Check sheet for the modelled part. Datum: model origin and axes. Units: mm. A direction names the side the tool comes from. Give positions to 0.01 mm unless a question says otherwise; leave off trailing zeros. Order: outer loops, then holes, each group sorted by start corner. A loop starts at its lowest first (then second) coordinate and runs counter-clockwise, first axis right, second up.
Item 1: Access from +Z, -Z, +X, -X, +Y, -Y to the whole of each face (thin tool, end or side, straight path). Record for faces 4 (the flat face through (7.5, 4.8, 0.7)), 5 (the flat face through (-3, 3, 0)), 6 (the flat face through (0, 8, -50)), 7 (the flat face through (0, 14, 10)), 8 (the flat face through (-5, 5, -1)).
Item 2: Sectioned sample at A-A on z = -23.5. Record the boundary of the cut face in (x, y), and give its area (3 significant figures).
Item 3: Gauge pin test, flat end, axial feed: P1, Ø7, axis at x = 0, z = 0, coming from the +Y side. Record the tip position at first contact, or that the pin passes through.
Item 4: Release check for a two-part mould opening along Z. For faces 1 (the flat face through (3, 0, 1)), 2 (the flat face through (0, 15, -10)), 3 (the flat face through (-0.1, 1.3, 48.8)) record: released by +Z, released by -Z, zero draft, split by the parting line, or undercut.
Item 5: Sectioned sample at D-D on z = 0. Record the boundary of the cut face in (x, y), and give its area (3 significant figures).
Item 6: Material ranges on line 1 along Y through (x, z) = (-1, 30); line 2 along Z through (x, y) = (0.75, 7.5); line 3 along Z through (x, y) = (1, 13.25), recorded low to high.
Item 7: Sectioned sample at B-B on y = 15.75. Record the boundary of the cut face in (x, z), and give its area (3 significant figures).
Item 8: Sectioned sample at C-C on x = 0. Record the boundary of the cut face in (y, z), and give its area (4 significant figures).
from build123d import *

# Parameters (mm, degrees)
BOSS_EXTRUDE1_DEPTH = 7.5
CHAMFER1_SIZE       = 2.5
SKETCH2_R           = 2.75
CUT_EXTRUDE1_DEPTH  = 52.963929798
SKETCH3_R           = 4.25
CUT_EXTRUDE2_DEPTH  = 2


with BuildPart() as part:
    # Sketch1 → Boss-Extrude1 (new, symmetric)
    with BuildSketch(Plane(origin=(0, 0, 0), x_dir=(0, 0, -1), z_dir=(1, 0, 0))):
        Polygon((10, 17), (10, 12), (45, 12), (45, 5), (-45, 5), (-45, 12), (-10, 12), (-10, 17), (-50, 17), (-50, 0), (50, 0), (50, 17), align=None)
    extrude(amount=BOSS_EXTRUDE1_DEPTH, both=True)

    # Chamfer1
    chamfer1_edges = [part.edges().sort_by_distance(p)[0] for p in [
        (0, 17, -50),
        (0, 0, -50),
        (0, 0, 50),
        (0, 17, 50),
        (0, 12, 45),
        (0, 5, 45),
        (0, 5, -45),
        (0, 12, -45),
    ]]
    chamfer(chamfer1_edges, length=CHAMFER1_SIZE)

    # Sketch2 → Cut-Extrude1 (cut, through all)
    with BuildSketch(Plane(origin=(0, 5, 0), x_dir=(1, 0, 0), z_dir=(0, 1, 0))):
        with Locations(Location((0, 0, 0), (0, 0, 270))):
            Circle(SKETCH2_R)
    extrude(amount=-CUT_EXTRUDE1_DEPTH, mode=Mode.SUBTRACT)

    # Sketch3 → Cut-Extrude2 (cut)
    with BuildSketch(Plane(origin=(0, 5, 0), x_dir=(1, 0, 0), z_dir=(0, 1, 0))):
        with Locations(Location((0, 0, 0), (0, 0, 270))):
            Circle(SKETCH3_R)
    extrude(amount=-CUT_EXTRUDE2_DEPTH, mode=Mode.SUBTRACT)


solid = part.part
Report:
1. face 4: +Z, -Z, +X, +Y, -Y
1. face 5: +Y
1. face 6: -Z, +X, -X, +Y, -Y
1. face 7: +X, -X, +Y
1. face 8: +X, -X
2. outline: (-7.5, 0) - (7.5, 0) - (7.5, 5) - (-7.5, 5) - close; (-7.5, 12) - (7.5, 12) - (7.5, 17) - (-7.5, 17) - close
2. area: 150 mm2
3. P1: stops at y = 3
4. face 1: zero draft
4. face 2: undercut
4. face 3: released by +Z
5. outline: (-7.5, 0) - (-2.75, 0) - (-2.75, 3) - (-4.25, 3) - (-4.25, 5) - (-7.5, 5) - close; (2.75, 0) - (7.5, 0) - (7.5, 5) - (4.25, 5) - (4.25, 3) - (2.75, 3) - close
5. area: 41.5 mm2
6. line 1: y = 0 to 5, 12 to 17
6. line 2: z = -50 to -45, 45 to 50
6. line 3: z = -50 to -10, 10 to 50
7. outline: (-7.5, -48.75) - (7.5, -48.75) - (7.5, -10) - (-7.5, -10) - close; (-7.5, 10) - (7.5, 10) - (7.5, 48.75) - (-7.5, 48.75) - close
7. area: 1,160 mm2
8. outline: (0, -47.5) - (2.5, -50) - (14.5, -50) - (17, -47.5) - (17, -10) - (12, -10) - (12, -42.5) - (9.5, -45) - (7.5, -45) - (5, -42.5) - (5, -4.25) - (3, -4.25) - (3, -2.75) - (0, -2.75) - close; (0, 2.75) - (3, 2.75) - (3, 4.25) - (5, 4.25) - (5, 42.5) - (7.5, 45) - (9.5, 45) - (12, 42.5) - (12, 10) - (17, 10) - (17, 47.5) - (14.5, 50) - (2.5, 50) - (0, 47.5) - close
8. area: 936.5 mm2
